Part model, mm, in its own coordinate system. A direction names the side the tool comes from. Coordinates: 2 decimals unless noted, no trailing zeros. Loops run counter-clockwise (first coordinate to the right, second up) from the corner with the lowest first, then second, coordinate; pieces in that order, holes last. Notation, with made-up numbers: M -11,56.5 L 13,56.5 A12 cw 13,75.5 Z; hole C -11,67 d9. An arc over 180 degrees is marked long. Answer as a JSON object with one key per item and string values. Group by question number.
1. Saw through at A-A on x = 0. Write the cut outline in (y, z) (3 decimals).
2. Saw through at D-D on y = 36. Write the cut outline in (x, z).
3. Drop flat-ended pins along their axis: pin 1 Ø8 at (x, z) = (-5.5, 8) entering from +Y; pin 2 Ø1.5 at (x, z) = (-23.5, 13) entering from +Y; pin 3 Ø2 at (y, z) = (57.5, -8) entering from -X; pin 4 Ø1.5 at (x, y) = (-6.5, 17.5) entering from -Z. Give the stop position or say it passes through.
4. 3-axis set-ups, long thin cutter, end or side, ignore diameter. For faces 1 (the face through (0, 26, -27.306)), 2 (the face through (-13, 20.32, -23)), 3 (the face through (22, 32.766, 13)), 4 (the face through (26, 20.32, 0)): which of +Z, -Z, +X, -X, +Y, -Y reach the whole face in a straight line?
5. Drill centre lines: L1, parallel to Z at x = 0, y = 13.5 (3 decimals); L2, parallel to Z at x = 0, y = 55; L3, parallel to Y at x = 15, z = -12. Where is each one in solid material? Low to high.
6. Saw through at B-B on z = -6. Write the cut outline in (x, y).
7. Mould opens along Z. For faces 5 (the face through (-11.5, 20.32, -13.1)), 6 (the face through (17.74, 45.95, -13.6)), 7 (the face through (-26, 20.32, 0)), 8 (the face through (-23.669, 26.456, 13.617)) say: released by +Z, released by -Z, zero draft, split by the parting line, or undercut.
8. Saw through at C-C on y = 7. Write the cut outline in (x, z) (3 decimals).
from build123d import *

# Parameters (mm, degrees)
SKETCH2_R           = 20.828
BASE_EXTRUDE_DEPTH  = 17.78
SKETCH3_R           = 27.4701
BOSS_EXTRUDE1_DEPTH = 2.54
BOSS_EXTRUDE3_DEPTH = 12.446
SKETCH6_R           = 25.146
BOSS_EXTRUDE4_DEPTH = 38.1
SKETCH7_R           = 22.352
CUT_EXTRUDE1_DEPTH  = 50.546
SKETCH8_R           = 17.145
CUT_EXTRUDE2_DEPTH  = 71.866


with BuildPart() as part:
    # Sketch2 → Base-Extrude (new body)
    with BuildSketch(Plane(origin=(0, 0, 0), x_dir=(1, 0, 0), z_dir=(0, 1, 0))):
        Circle(SKETCH2_R)
    extrude(amount=BASE_EXTRUDE_DEPTH)

    # Sketch3 → Boss-Extrude1 (add)
    with BuildSketch(Plane(origin=(0, 17.78, 0), x_dir=(-1, 0, 0), z_dir=(0, 1, 0))):
        Circle(SKETCH3_R)
    extrude(amount=BOSS_EXTRUDE1_DEPTH)

    # Sketch5 → Boss-Extrude3 (add)
    with BuildSketch(Plane(origin=(0, 20.32, 0), x_dir=(-1, 0, 0), z_dir=(0, 1, 0))):
        Polygon((25.146, -11.058258362), (25.146, 11.058258362), (22.149732663, 16.247945622), (2.996267337, 27.306203985), (-2.996267337, 27.306203985), (-22.149732663, 16.247945622), (-25.146, 11.058258362), (-25.146, -11.058258362), (-22.149732663, -16.247945622), (-2.996267337, -27.306203985), (2.996267337, -27.306203985), (22.149732663, -16.247945622), align=None)
    extrude(amount=BOSS_EXTRUDE3_DEPTH)

    # Sketch6 → Boss-Extrude4 (add)
    with BuildSketch(Plane(origin=(0, 32.766, 0), x_dir=(-1, 0, 0), z_dir=(0, 1, 0))):
        Circle(SKETCH6_R)
    extrude(amount=BOSS_EXTRUDE4_DEPTH)

    # Sketch7 → Cut-Extrude1 (cut)
    with BuildSketch(Plane(origin=(0, 70.866, 0), x_dir=(-1, 0, 0), z_dir=(0, 1, 0))):
        Circle(SKETCH7_R)
    extrude(amount=-CUT_EXTRUDE1_DEPTH, mode=Mode.SUBTRACT)

    # Sketch8 → Cut-Extrude2 (cut, through all)
    with BuildSketch(Plane.XZ):
        Circle(SKETCH8_R)
    extrude(amount=-CUT_EXTRUDE2_DEPTH, mode=Mode.SUBTRACT)


solid = part.part
Outcome:
{
 "1": {"outline": "M 0,-20.828 L 17.78,-20.828 L 17.78,-27.47 L 20.32,-27.47 L 20.32,-27.306 L 32.766,-27.306 L 32.766,-25.146 L 70.866,-25.146 L 70.866,-22.352 L 20.32,-22.352 L 20.32,-17.145 L 0,-17.145 Z; M 0,17.145 L 20.32,17.145 L 20.32,22.352 L 70.866,22.352 L 70.866,25.146 L 32.766,25.146 L 32.766,27.306 L 20.32,27.306 L 20.32,27.47 L 17.78,27.47 L 17.78,20.828 L 0,20.828 Z"},
 "2": {"outline": "C 0,0 d50.29; hole C 0,0 d44.7"},
 "3": {"pin 1": "passes through", "pin 2": "stops at y = 32.77", "pin 3": "stops at x = -24.15", "pin 4": "stops at z = -26.85"},
 "4": {"face 1": "-Z, +X, -X, +Y", "face 2": "-Z, -X, +Y", "face 3": "+Z, +X, +Y", "face 4": "+Z, -Z, +X, +Y"},
 "5": {"L1": "z = -20.828 to -17.145, 17.145 to 20.828", "L2": "z = -25.15 to -22.35, 22.35 to 25.15", "L3": "y = 0 to 20.32"},
 "6": {"outline": "M -26.81,17.78 L -19.95,17.78 L -19.95,0 L -16.06,0 L -16.06,20.32 L -21.53,20.32 L -21.53,70.87 L -24.42,70.87 L -24.42,32.77 L -25.15,32.77 L -25.15,20.32 L -26.81,20.32 Z; M 16.06,0 L 19.95,0 L 19.95,17.78 L 26.81,17.78 L 26.81,20.32 L 25.15,20.32 L 25.15,32.77 L 24.42,32.77 L 24.42,70.87 L 21.53,70.87 L 21.53,20.32 L 16.06,20.32 Z"},
 "7": {"face 5": "undercut", "face 6": "undercut", "face 7": "zero draft", "face 8": "released by +Z"},
 "8": {"outline": "C 0,0 d41.656; hole C 0,0 d34.29"}
}
